Geometry check sheet. Reference: the model listing, model coordinates, mm. A direction names the side the tool comes from. Round coordinates to 2 decimals unless told otherwise and drop trailing zeros. Order: outer loops, then holes, each group sorted by start corner. A loop starts at its lowest first (then second) coordinate and runs counter-clockwise, first axis right, second up.
(1) Gauge pin test, flat ends, axial feed: P1, Ø12, axis at y = 21.5, z = -15.5, coming from the +X side; P2, Ø2, axis at x = 29, y = 17.5, coming from the -Z side; P3, Ø2.5, axis at x = -6.35, z = -9.525, coming from the -Y side; P4, Ø6.5, axis at x = -9.5, z = -49.5, coming from the +Y side. Record the tip position at first contact, or that the pin passes through.
(2) Set-up check for faces 1 (the face through (-4.206, 0.258, -10.2)), 2 (the face through (-6, 0.508, -35)): record each of +Z, -Z, +X, -X, +Y, -Y from which the full face is reachable in a straight line by a thin tool's end or side.
(3) Cross-section at D-D on y = 20.5. Enter the section's corners in (x, z).
(4) Cross-section at C-C on x = 26.5. Enter the section's corners in (y, z), and give its area (3 significant figures).
(5) Cross-section at A-A on x = -6.35. Enter the section's corners in (y, z).
(6) Thickness scan on L1, parallel to Z at x = -6.35, y = 0.4; L2, parallel to Y at x = -6, z = -65.5; L3, parallel to Y at x = 18, z = -12. Record the ranges inside material, lowest first.
from build123d import *

# Parameters (mm, degrees)
SKETCH2_W             = 12.7
SKETCH2_H             = 69.85
BOSS_EXTRUDE2_DEPTH   = 0.508
EDGE_FLANGE2_DEPTH    = 69.85
F_8_CLEARANCE_HOLE1_D = 4.4958


# Sheet-metal steps are written as plain solids
with BuildPart() as part:
    # Sketch2 → Boss-Extrude2 (new body)
    with BuildSketch(Plane(origin=(0, 0, 0), x_dir=(1, 0, 0), z_dir=(0, 1, 0))):
        with Locations((-6.35, 34.925)):
            Rectangle(SKETCH2_W, SKETCH2_H)
    extrude(amount=BOSS_EXTRUDE2_DEPTH)

    # Edge-Flange2 section (across the edge) → Edge-Flange2 (add)
    with BuildSketch(Plane(origin=(0.850738686, 0.508, 0), x_dir=(-0.49999999999999495, 0.8660254037844416, 0), z_dir=(0, 0, -1))):
        with BuildLine():
            Line((-0.508, 0.850738686), (-0.508, 56.2102))
            Line((-0.508, 56.2102), (0, 56.2102))
            Line((0, 56.2102), (0, 0.850738686))
            ThreePointArc((0, 0.850738686), (0.108185502, 0.028988218), (0.425369343, -0.736761314))
            Line((0.425369343, -0.736761314), (-0.014571562, -0.990761314))
            ThreePointArc((-0.014571562, -0.990761314), (-0.382504818, -0.102491857), (-0.508, 0.850738686))
        make_face()
    extrude(amount=EDGE_FLANGE2_DEPTH)

    # #8 Clearance Hole1 (through all)
    with Locations(Plane(origin=(0, 0, 0), x_dir=(-1, 0, 0), z_dir=(0, -1, 0))):
        with Locations((6.35, 60.325), (6.35, 9.525)):
            Hole(F_8_CLEARANCE_HOLE1_D / 2)


solid = part.part
Found:
1. P1: stops at x = 48.62
1. P2: stops at z = -69.85
1. P3: passes through
1. P4: stops at y = 0.51
2. face 1: +Y, -Y
2. face 2: +Z, -Z, -X, +Y
3. outline: (35.48, -69.85) - (36.49, -69.85) - (36.49, 0) - (35.48, 0) - close
4. outline: (14.73, -69.85) - (15.32, -69.85) - (15.32, 0) - (14.73, 0) - close
4. area: 41.0 mm2
5. outline: (0, -69.85) - (0.51, -69.85) - (0.51, -62.57) - (0, -62.57) - close; (0, -58.08) - (0.51, -58.08) - (0.51, -11.77) - (0, -11.77) - close; (0, -7.28) - (0.51, -7.28) - (0.51, 0) - (0, 0) - close
6. L1: z = -69.85 to -62.57, -58.08 to -11.77, -7.28 to 0
6. L2: y = 0 to 0.51
6. L3: y = 9.82 to 10.41
